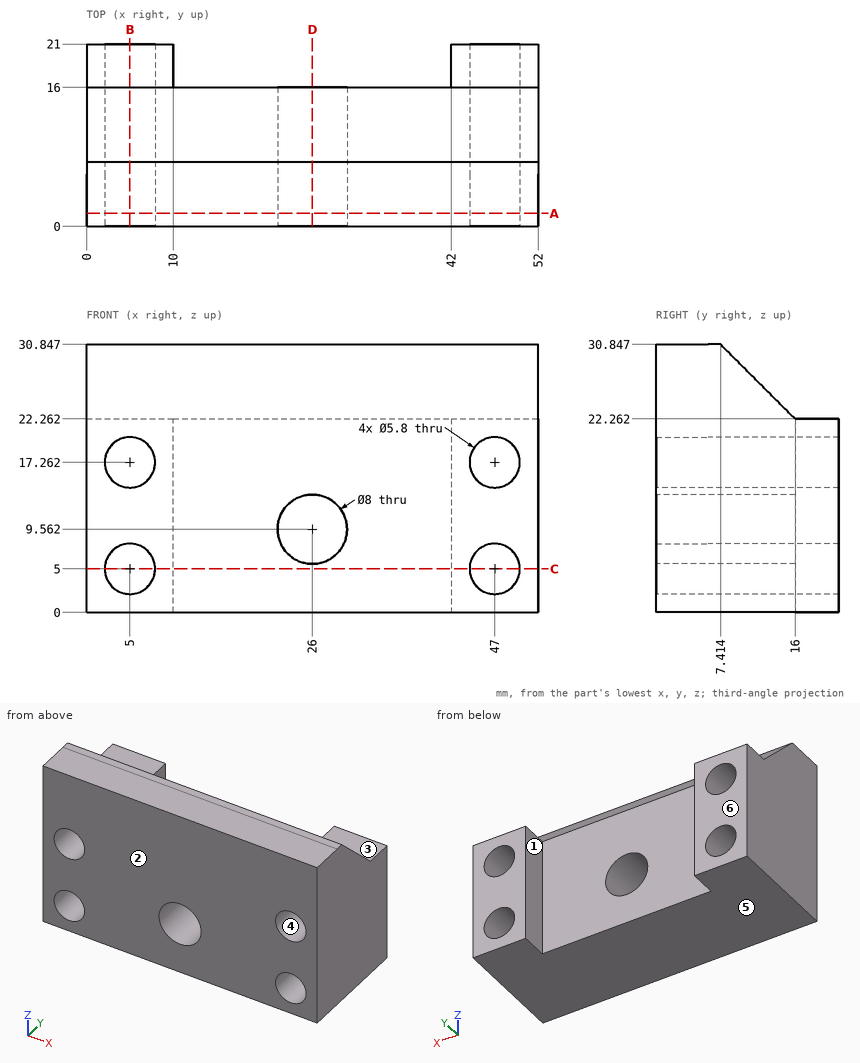
The drawing under review shows one solid part. Ordinate dimensions are in mm from its lowest x, y, z. A direction names the side the tool comes from. Round coordinates to 2 decimals unless told otherwise and drop trailing zeros. Write each loop counter-clockwise with the first axis right and the second up, starting at its lowest first coordinate (ties: lowest second). Pieces come first, ordered by that corner, then holes. Notation, with made-up numbers: (29, 85) - (41, 85) arc R20 cw to (41, 112) - close; hole circle Ø1 at (12.25, 61). An arc over 180 degrees is marked (long way). Write each question's results on one line, items separated by ' | '.
Item 1: Take a section at C-C on z = 5. State the section outline as (x, y) points.
Calculated:
outline: (0, 0) - (2.1, 0) - (2.1, 21) - (0, 21) - close; (7.9, 0) - (44.1, 0) - (44.1, 21) - (42, 21) - (42, 16) - (10, 16) - (10, 21) - (7.9, 21) - close; (49.9, 0) - (52, 0) - (52, 21) - (49.9, 21) - close
Item 2: Take a section at B-B on x = 5. State the section outline as (y, z) points (1 decimal).
Calculated:
outline: (0, 0) - (21, 0) - (21, 2.1) - (0, 2.1) - close; (0, 7.9) - (21, 7.9) - (21, 14.4) - (0, 14.4) - close; (0, 20.2) - (21, 20.2) - (21, 22.3) - (16, 22.3) - (7.4, 30.8) - (0, 30.8) - close
Item 3: For pin 1 (10 mm diameter, centred on x = 22, z = 23.5, fed in from +Y); pin 2 (2.5 mm diameter, centred on x = 2.5, y = 19, fed in from +Z), all flat-tipped, find the tip position at first contact; note any pin that passes through.
Calculated:
pin 1: stops at y = 16 | pin 2: stops at z = 22.26
Item 4: Take a section at A-A on y = 1.5. State the section outline as (x, z) points.
Calculated:
outline: (0, 0) - (52, 0) - (52, 30.85) - (0, 30.85) - close; hole circle Ø5.8 at (5, 5); hole circle Ø5.8 at (5, 17.26); hole circle Ø8 at (26, 9.56); hole circle Ø5.8 at (47, 5); hole circle Ø5.8 at (47, 17.26)
Item 5: To check wall thickness, follow line 1 along Z through (x, y) = (5, 4.5); line 2 along Z through (x, y) = (47, 16.75); line 3 along X through (y, z) = (18.75, 21.5). State the ranges of each line that lie inside material, in increasing order. Write a range as from..to.
Calculated:
line 1: z = 0..2.1, 7.9..14.36, 20.16..30.85 | line 2: z = 0..2.1, 7.9..14.36, 20.16..22.26 | line 3: x = 0..10, 42..52
Item 6: Draft analysis for pull direction Z (two halves, no side actions). For the marked faces 4, 5 and 6, state which applies: pulls with the +Z half, pulls with the -Z half, needs draft (parallel to the pull), parting line crosses it, or undercut.
Calculated:
face 4: undercut | face 5: pulls with the -Z half | face 6: needs draft
Item 7: Take a section at D-D on x = 26. State the section outline as (y, z) points (1 decimal).
Calculated:
outline: (0, 0) - (16, 0) - (16, 5.6) - (0, 5.6) - close; (0, 13.6) - (16, 13.6) - (16, 22.3) - (7.4, 30.8) - (0, 30.8) - close
Item 8: For the marked faces 1, 2 and 3, list the 3-axis set-ups (+Z, -Z, +X, -X, +Y, -Y) from which the entire face can be reached by the end or side of a thin tool; tool diameter is ignored.
Calculated:
face 1: +Z, -Z, +Y | face 2: +Z, -Z, +X, -X, -Y | face 3: +Z, +X, -X, +Y
